Answer from the drawing. Dimensions are ordinates in mm from the lowest x, y and z of the part. Give positions to 0.01 mm unless a question says otherwise; leave off trailing zeros. Order: outer loops, then holes, each group sorted by start corner. A loop starts at its lowest first (then second) coordinate and runs counter-clockwise, first axis right, second up. Notation, with made-up numbers: (-11, 40.5) -> (31, 40.5) arc R6 ccw to (31, 46.5) -> close; hole circle Ø3 at (5.5, -4). An arc over 180 degrees is marked (long way). Answer as a JSON object with one key per item and string values. Group by question number.
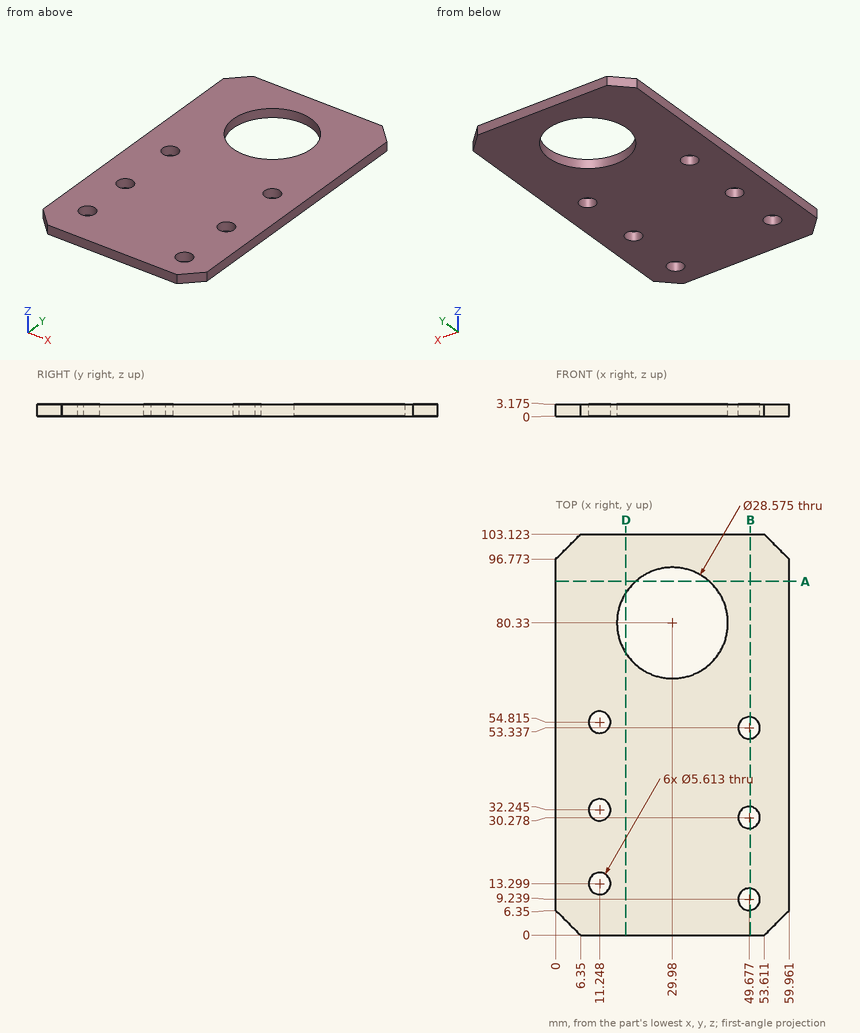
(1) Find the intervals of material crossed by line 1 along Y through (x, z) = (13.5, 0.85) (1 decimal); line 2 along X through (y, z) = (53.5, 1.8) (1 decimal); line 3 along X through (y, z) = (68.5, 1.25) (1 decimal), in increasing order. Write a range as [from, to].
(2) A cutting plane is placed at B-B (x = 50). State how many separate pieces and enclosed holes the cut face has, and give its area (3 significant figures).
(3) A cutting plane is placed at D-D (x = 18). Determine the outline of the cut face in (y, z) (1 decimal), and give its area (3 significant figures).
(4) A cutting plane is placed at A-A (y = 91). Determine the outline of the cut face in (x, z) (1 decimal), and give its area (3 significant figures).
(5) A flat-ended cylindrical pin translates along its axis: pin 1 Ø7.5 at (x, y) = (11.25, 13.3) entering from +Z (1 decimal). Find the tip coordinate at first contact, or state that the pin passes through.
Check sheet entries:
{
 "1": {"line 1": "y = [0, 11.6], [15, 30.6], [33.9, 53.1], [56.5, 103.1]", "line 2": "x = [0, 8.8], [13.7, 46.9], [52.5, 60]", "line 3": "x = [0, 22], [38, 60]"},
 "2": {"separate pieces": "4", "enclosed holes": "0", "area": "274 mm2"},
 "3": {"outline": "(0, 0) -> (72.5, 0) -> (72.5, 3.2) -> (0, 3.2) -> close; (88.1, 0) -> (103.1, 0) -> (103.1, 3.2) -> (88.1, 3.2) -> close", "area": "278 mm2"},
 "4": {"outline": "(0, 0) -> (20.5, 0) -> (20.5, 3.2) -> (0, 3.2) -> close; (39.5, 0) -> (60, 0) -> (60, 3.2) -> (39.5, 3.2) -> close", "area": "130 mm2"},
 "5": {"pin 1": "stops at z = 3.2"}
}
